Geometry: final body of the model. Coordinates: model frame, mm. Face numbers are marked on the shaded views. A direction names the side the tool comes from. Give positions to 0.01 mm unless a question says otherwise; leave off trailing zeros. Write each loop counter-clockwise with the first axis right and the second up, starting at its lowest first coordinate (ties: lowest second). Pieces come first, ordered by that corner, then holes. Notation, with made-up numbers: (2, 37.5) -> (61, 37.5) arc R18 ccw to (61, 72.5) -> close; hole circle Ø7 at (-36, 30). An arc over 180 degrees is marked (long way). Answer in a Markdown table with one row per item. Add a question column.
Item 1: Section query D-D on x = 0. Output: boundary loops of the cut face in (y, z) (3 decimals), plus the area to 3 significant figures.
Item 2: Access query for the marked faces 5, 6 and 7. Directions: +Z, -Z, +X, -X, +Y, -Y. A direction counts if a zero-diameter tool reaches every point of the face in a straight line with its end or side. Return the directions, or none.
Item 3: Material intervals for probe 1 along X at (y, z) = (7, -6.25); probe 2 along Z at (x, y) = (29.21, 1.6) (3 decimals); probe 3 along Z at (x, y) = (29.21, 8.5) (3 decimals), sorted ascending. Write a range as from..to.
Item 4: Section query A-A on y = 6.5. State how many separate pieces and enclosed holes the cut face has, plus the area to 3 significant figures.
Item 5: Draft query along Z for the marked faces 1, 2, 3 and 4. Return one class per face: +Z half, -Z half, draft (parallel to the pull), parting line (faces both ways), or undercut.
Item 6: First-contact query: P1, Ø5, axis at x = 2.5, z = 7, coming from the -Y side; P2, Ø1.5, axis at y = 19.5, z = 0, coming from the +X side; P3, Ø5.5, axis at x = 29.21, z = 0, coming from the -Y side; P4, Ø4, axis at x = 23, z = -1.5, coming from the +Y side. Flat tips, straight axial feed; report the tip coordinate or a pass-through.
```python
from build123d import *

# Parameters (mm, degrees)
BOSS_EXTRUDE1_DEPTH                                  = 9.525
BOSS_EXTRUDE2_DEPTH                                  = 9.525
FILLET1_R                                            = 3.175
CBORE_FOR_1_4_BINDING_HEAD_MACHINE_SCREW_D           = 6.7564
CBORE_FOR_1_4_BINDING_HEAD_MACHINE_SCREW_CBORE_D     = 14.2875
CBORE_FOR_1_4_BINDING_HEAD_MACHINE_SCREW_CBORE_DEPTH = 4.191


with BuildPart() as part:
    # Sketch1 → Boss-Extrude1 (new, symmetric)
    with BuildSketch(Plane.XY):
        with BuildLine():
            Line((-22.225, 0), (-12.7, 0))
            ThreePointArc((-12.7, 0), (0, 12.7), (12.7, 0))
            Line((12.7, 0), (22.225, 0))
            ThreePointArc((22.225, 0), (0, 22.225), (-22.225, 0))
        make_face()
    extrude(amount=BOSS_EXTRUDE1_DEPTH, both=True)

    # Sketch2 → Boss-Extrude2 (add)
    with BuildSketch(Plane.XZ):
        with BuildLine():
            Line((-12.7, -9.525), (-29.21, -9.525))
            ThreePointArc((-29.21, -9.525), (-38.735, 0), (-29.21, 9.525))
            Line((-29.21, 9.525), (-12.7, 9.525))
            Line((-12.7, 9.525), (-12.7, -9.525))
        make_face()
        with BuildLine():
            Line((12.7, 9.525), (12.7, -9.525))
            Line((12.7, -9.525), (29.21, -9.525))
            ThreePointArc((29.21, -9.525), (38.735, 0), (29.21, 9.525))
            Line((29.21, 9.525), (12.7, 9.525))
        make_face()
    extrude(amount=-BOSS_EXTRUDE2_DEPTH)

    # Fillet1
    fillet1_edges = [part.edges().sort_by_distance(p)[0] for p in [
        (-20.080463142, 9.525, 0),
        (20.080463142, 9.525, 0),
    ]]
    fillet(fillet1_edges, radius=FILLET1_R)

    # CBORE for 1/4 Binding Head Machine Screw1 (through all)
    with Locations(Plane(origin=(0, 9.525, 0), x_dir=(1, 0, 0), z_dir=(0, 1, 0))):
        with Locations((-29.21, 0), (29.21, 0)):
            CounterBoreHole(CBORE_FOR_1_4_BINDING_HEAD_MACHINE_SCREW_D / 2, CBORE_FOR_1_4_BINDING_HEAD_MACHINE_SCREW_CBORE_D / 2, CBORE_FOR_1_4_BINDING_HEAD_MACHINE_SCREW_CBORE_DEPTH)


solid = part.part
```
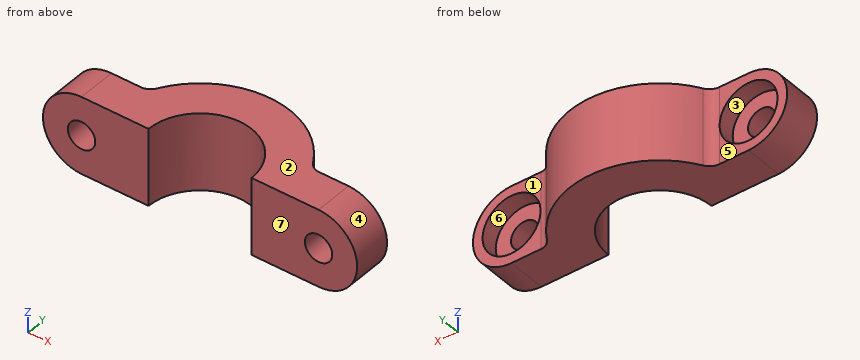
Findings below:
| question | item | result |
|---|---|---|
| 1 | outline | (12.7, -9.525) -> (22.225, -9.525) -> (22.225, 9.525) -> (12.7, 9.525) -> close |
| 1 | area | 181 mm^2 |
| 2 | face 5 | +Z, -Z, -X, +Y |
| 2 | face 6 | +Y |
| 2 | face 7 | +Z, -Z, +X, -X, -Y |
| 3 | probe 1 | x = -36.4..-32.67, -25.75..-10.6, 10.6..25.75, 32.67..36.4 |
| 3 | probe 2 | z = -9.525..-3.378, 3.378..9.525 |
| 3 | probe 3 | z = -9.525..-7.144, 7.144..9.525 |
| 4 | separate pieces | 2 |
| 4 | enclosed holes | 2 |
| 4 | area | 662 mm^2 |
| 5 | face 1 | draft |
| 5 | face 2 | +Z half |
| 5 | face 3 | undercut |
| 5 | face 4 | parting line |
| 6 | P1 | stops at y = 11.67 |
| 6 | P2 | stops at x = 11.93 |
| 6 | P3 | passes through |
| 6 | P4 | stops at y = 9.69 |
